The listing builds one solid part. Answer for the finished solid, in the listing's coordinates (mm). A direction names the side the tool comes from. Give positions to 0.01 mm unless a question says otherwise; leave off trailing zeros. Order: outer loops, then holes, each group sorted by start corner. A loop starts at its lowest first (then second) coordinate and runs counter-clockwise, first axis right, second up. Notation, with made-up numbers: (-12, 50.5) - (26, 50.5) arc R11 ccw to (26, 56.5) - close; hole circle Ø6 at (-27, 17). An arc over 180 degrees is marked (long way). Use a Markdown table: item, result. Add a question column.
1) Find section A-A, the plane x = 654.5. Determine the outline of the cut face in (y, z) (3 decimals).
2) Find section B-B, the plane y = 2.6. State how many separate pieces and enclosed holes the cut face has, plus the area to 3 significant figures.
3) Straight lines are drawn through the part: line 1 (Z direction, x = 253, y = 1.7); line 2 (X direction, y = 2.95, z = 496.5); line 3 (Z direction, x = 243, y = 1.6). For each, find the intervals that lie inside material, in ascending order.
4) Flat-ended cylindrical pins translate along their axes: pin 1 (1 mm diameter, centred on x = 266.5, y = 1, fed in from +Z); pin 2 (6.5 mm diameter, centred on x = 565.76, z = 565.76, fed in from -Y) (3 decimals); pin 3 (1.5 mm diameter, centred on x = 229, y = 2.5, fed in from +Z). Find the tip coordinate at first contact, or state that the pin passes through.
5) For faces 1 (the face through (456.76, 1.57, 398.39)), 2 (the face through (158.171, 1.565, 536.482)), determine the directions among +Z, -Z, +X, -X, +Y, -Y from which every point of the face is accessible in a straight line to the end or side of a thin tool.
6) The mould has two halves that part along X. Classify faces 3 (the face through (238.34, 1.57, 584.07)), 4 (the face through (794.12, 1.57, 123.44)), 5 (the face through (274.942, 1.565, 468.953)): released by +X, released by -X, zero draft, split by the parting line, or undercut.
from build123d import *

# Parameters (mm, degrees)
BOSS_EXTRUDE1_DEPTH         = 3.175
FILLET3_R                   = 38.1
F_5_16_0_3125_DOWEL_HOLE1_D = 7.9375
F_1_2_DOWEL_SLOT1_DEPTH     = 3.175
FILLET4_R                   = 25.4
FILLET6_R                   = 12.7


# Read off the part's stored shape, not the designer's step: 1 (2) Dowel Slot1
with BuildPart() as part:
    # Sketch1 → Boss-Extrude1 (new body)
    with BuildSketch(Plane(origin=(0, 0, 0), x_dir=(1, 0, 0), z_dir=(0, 1, 0))):
        Polygon((246.957043329, -947.417020773), (947.417020773, -246.957043329), (911.495996289, -211.036018845), (808.524005584, -163.019391004), (776.924331502, -76.2), (552.45, -76.2), (552.45, -114.3), (521.073488184, -200.506257716), (413.091781569, -354.720116782), (502.89434278, -444.522677993), (444.522677993, -502.89434278), (354.720116782, -413.091781569), (200.506257716, -521.073488184), (114.3, -552.45), (76.2, -552.45), (76.2, -776.924331502), (163.019391004, -808.524005584), (211.036018845, -911.495996289), align=None)
    extrude(amount=BOSS_EXTRUDE1_DEPTH)

    # Fillet3
    fillet3_edges = [part.edges().sort_by_distance(p)[0] for p in [
        (76.2, 1.5875, 552.45),
        (552.45, 1.5875, 76.2),
    ]]
    fillet(fillet3_edges, radius=FILLET3_R - 0.0001)  # a hair under: the kernel refuses the full size

    # 5/16 (0.3125) Dowel Hole1 (through all)
    with Locations(Plane(origin=(0, 3.175, 0), x_dir=(1, 0, 0), z_dir=(0, 1, 0))):
        with Locations((252.197410095, -508.134709545), (508.134709545, -252.197410095), (902.515740167, -228.996531087), (228.996531087, -902.515740167), (565.756135627, -565.756135627)):
            Hole(F_5_16_0_3125_DOWEL_HOLE1_D / 2)

    # 1 (2) Dowel Slot1 outline → 1 (2) Dowel Slot1 (cut)
    with BuildSketch(Plane(origin=(0, 0, 0), x_dir=(1, 0, 0), z_dir=(0, 1, 0))):
        with BuildLine():
            Line((530.585349848, -328.529587124), (584.466886574, -274.648050397))
            ThreePointArc((584.466886574, -274.648050397), (584.466886574, -238.727025913), (548.54586209, -238.727025913))
            Line((548.54586209, -238.727025913), (494.664325364, -292.60856264))
            ThreePointArc((494.664325364, -292.60856264), (494.664325364, -328.529587124), (530.585349848, -328.529587124))
        make_face()
        with BuildLine():
            ThreePointArc((328.529587124, -530.585349848), (328.529587124, -494.664325364), (292.60856264, -494.664325364))
            Line((292.60856264, -494.664325364), (238.727025913, -548.54586209))
            ThreePointArc((238.727025913, -548.54586209), (238.727025913, -584.466886574), (274.648050397, -584.466886574))
            Line((274.648050397, -584.466886574), (328.529587124, -530.585349848))
        make_face()
    extrude(amount=F_1_2_DOWEL_SLOT1_DEPTH, mode=Mode.SUBTRACT)

    # Fillet4
    fillet4_edges = [part.edges().sort_by_distance(p)[0] for p in [
        (211.036018845, 1.5875, 911.495996289),
        (163.019391004, 1.5875, 808.524005584),
        (76.2, 1.5875, 776.924331502),
        (776.924331502, 1.5875, 76.2),
        (808.524005584, 1.5875, 163.019391004),
        (911.495996289, 1.5875, 211.036018845),
    ]]
    fillet(fillet4_edges, radius=FILLET4_R)

    # Fillet6
    fillet6_edges = [part.edges().sort_by_distance(p)[0] for p in [
        (947.417020773, 1.5875, 246.957043329),
        (246.957043329, 1.5875, 947.417020773),
        (114.3, 1.5875, 552.45),
        (200.506257716, 1.5875, 521.073488184),
        (354.720116782, 1.5875, 413.091781569),
        (444.522677993, 1.5875, 502.89434278),
        (502.89434278, 1.5875, 444.522677993),
        (413.091781569, 1.5875, 354.720116782),
        (521.073488184, 1.5875, 200.506257716),
        (552.45, 1.5875, 114.3),
    ]]
    fillet(fillet6_edges, radius=FILLET6_R)


solid = part.part
The answers:
| question | item | result |
|---|---|---|
| 1 | outline | (0, 76.2) - (3.175, 76.2) - (3.175, 539.874) - (0, 539.874) - close |
| 2 | separate pieces | 1 |
| 2 | enclosed holes | 7 |
| 2 | area | 293,000 mm2 |
| 3 | line 1 | 484.32 to 504.25, 512.02 to 534.27, 591.64 to 940.63 |
| 3 | line 2 | 235.6 to 290.77, 330.19 to 439.28, 449.77 to 697.87 |
| 3 | line 3 | 491.32 to 544.27, 587.9 to 941.52 |
| 4 | pin 1 | z = 928.37 |
| 4 | pin 2 | through |
| 4 | pin 3 | z = 930.21 |
| 5 | face 1 | +Y, -Y |
| 5 | face 2 | -Z, -X, +Y, -Y |
| 6 | face 3 | undercut |
| 6 | face 4 | released by +X |
| 6 | face 5 | released by -X |
